Autodesk Inventor part; units mm, degrees
ref_plane "YZ Plane" through (0, 0, 0) normal (1, 0, 0) x (0, 1, 0)
ref_plane "XZ Plane" through (0, 0, 0) normal (0, 1, 0) x (-1, 0, 0)
ref_plane "XY Plane" through (0, 0, 0) normal (0, 0, 1) x (1, 0, 0)
sketch "Esboço1" plane through (0, 0, 0) normal (0, 1, 0) x (-1, 0, 0)
  line L0 (0, 0) -> (-91, 0)
  line L1 (-91, 0) -> (-91, -111)
  line L2 (-91, -111) -> (0, -111)
  line L3 (0, -111) -> (0, 0)
  line L4 (-3, -108) -> (-88, -108)
  line L5 (-88, -108) -> (-88, -3)
  line L6 (-88, -3) -> (-3, -3)
  line L7 (-3, -3) -> (-3, -108)
  dimension "d0" = 3
  dimension "d1" = 3
  dimension "d2" = 3
  dimension "d3" = 3
  dimension "d4" = 85
  dimension "d5" = 105
extrude "Extrusão1" add sketch "Esboço1" along normal blind 3 contours L4 L5 L6 L7
extrude "Extrusão2" add sketch "Esboço1" along normal blind 25
sketch "Esboço2" plane through (0, 0, 0) normal (0, 0, 1) x (1, 0, 0)
  circle A0 centre (20, 12) radius 3
  circle A1 centre (66, 13) radius 3.75
  line L0 (0, 0) -> (0, 25)
  line L1 (91, 0) -> (91, 25)
  line L2 (0, 0) -> (91, 0)
  point P0 (0, 12.5)
  dimension "d10" = 6
  dimension "d11" = 7.5
  dimension "d25" = 20
  dimension "d26" = 25
  dimension "d30" = 13
  dimension "d31" = 12
extrude "Extrusão3" cut sketch "Esboço2" against normal blind 30
sketch "Esboço3" plane through (91, 0, 0) normal (1, 0, 0) x (0, 0, -1)
  circle A0 centre (16.1671, 10) radius 1.5
  circle A1 centre (34.0898, 10) radius 1.5
  circle A2 centre (25.3707, 10) radius 1.5
  line L0 (0, 0) -> (111, 0)
  dimension "d14" = 3
  dimension "d15" = 3
  dimension "d16" = 3
  dimension "d32" = 10
  dimension "d33" = 10
  dimension "d34" = 10
extrude "Extrusão4" cut sketch "Esboço3" against normal blind 10
sketch "Esboço4" plane through (0, 3, 0) normal (0, 1, 0) x (1, 0, 0)
  line L0 (28.1, 81.6) -> (63, 81.6)
  line L1 (63, 81.6) -> (63, 98)
  line L2 (63, 98) -> (28.1, 98)
  line L3 (28.1, 98) -> (28.1, 81.6)
  line L4 (88, 108) -> (88, 3)
  line L5 (3, 108) -> (88, 108)
  point P0 (0, 0)
  point P1 (63, 89.8)
  dimension "d19" = 34.9
  dimension "d20" = 16.4
  dimension "d23" = 25
  dimension "d24" = 10
extrude "Extrusão5" cut sketch "Esboço4" against normal blind 1.5
properties part number "Caixa_3DPrint"
Work out the finished part from the listing and answer in its coordinate system (mm). A direction names the side the tool comes from. Coordinates: 2 decimals unless noted, no trailing zeros. Loops run counter-clockwise (first coordinate to the right, second up) from the corner with the lowest first, then second, coordinate; pieces in that order, holes last. Notation, with made-up numbers: M -34.5,3 L -12.5,3 A30 cw -12.5,26 Z; hole C 52.5,35 d3. An arc over 180 degrees is marked long. Answer in a Markdown table with one row per item. Add a question column.
1. Find section B-B, the plane y = 18.25. Write down the section's boundary in (x, z), then the cut area to 3 significant figures.
2. Find section C-C, the plane z = -94. Write down the section's boundary in (x, y), then the cut area to 3 significant figures.
3. Find section A-A, the plane x = 20. Write down the section's boundary in (y, z), then the cut area to 3 significant figures.
4. A tool of negligible diameter and unlimited length cuts with its end or side. For faces 5 (the cylindrical face through (69.577, 14.126, -1.479)), 6 (the flat face through (46, 12, -111)), 7 (the flat face through (46, 3, -55)), 8 (the cylindrical face through (89.52, 10.45, -17.6)), 9 (the flat face through (90, 25, -55)), from which of +Z, -Z, +X, -X, +Y, -Y can it reach the whole face along a straight path? Write none if from no direction.
5. The mould has two halves that part along X. Classify faces 1 (the flat face through (45, 1.5, -90)), 2 (the flat face through (91, 12, -55)), 3 (the cylindrical face through (89.521, 10.066, -23.872)), 4 (the flat face through (3, 14, -55)): pulls with the +X half, pulls with the -X half, needs draft (parallel to the pull), parting line crosses it, or undercut.
6. Find section D-D, the plane x = 48. Write down the section's boundary in (y, z), then the cut area to 3 significant figures.
7. Flat-ended cylindrical pins translate along their axes: P1, Ø4.5, axis at x = 66, y = 13, coming from the +Z side; P2, Ø8, axis at x = 40.5, z = -90, coming from the +Y side; P3, Ø8, axis at x = 51.5, z = -83.5, coming from the +Y side. Find the tip coordinate at first contact, or state that the pin passes through.
8. Consider L1, parallel to X at y = 13, z = -23; L2, parallel to Z at x = 44.5, y = 15.5; L3, parallel to Y at x = 66, z = -0.7. Determine where each line is inside the solid, lowest interval first.
Reported:
| question | item | result |
|---|---|---|
| 1 | outline | M 0,-111 L 91,-111 L 91,0 L 0,0 Z; hole M 3,-108 L 88,-108 L 88,-3 L 3,-3 Z |
| 1 | area | 1,180 mm^2 |
| 2 | outline | M 0,0 L 91,0 L 91,25 L 88,25 L 88,3 L 63,3 L 63,1.5 L 28.1,1.5 L 28.1,3 L 3,3 L 3,25 L 0,25 Z |
| 2 | area | 353 mm^2 |
| 3 | outline | M 0,-111 L 25,-111 L 25,-108 L 3,-108 L 3,-3 L 9,-3 L 9,0 L 0,0 Z; M 15,-3 L 25,-3 L 25,0 L 15,0 Z |
| 3 | area | 447 mm^2 |
| 4 | face 5 | +Z |
| 4 | face 6 | -Z, +X, -X, +Y, -Y |
| 4 | face 7 | +Y |
| 4 | face 8 | +X |
| 4 | face 9 | +Z, -Z, +X, -X, +Y |
| 5 | face 1 | undercut |
| 5 | face 2 | pulls with the +X half |
| 5 | face 3 | needs draft |
| 5 | face 4 | undercut |
| 6 | outline | M 0,-111 L 25,-111 L 25,-108 L 3,-108 L 3,-98 L 1.5,-98 L 1.5,-81.6 L 3,-81.6 L 3,-3 L 25,-3 L 25,0 L 0,0 Z |
| 6 | area | 440 mm^2 |
| 7 | P1 | stops at z = -108 |
| 7 | P2 | stops at y = 1.5 |
| 7 | P3 | stops at y = 3 |
| 8 | L1 | x = 0 to 3, 88 to 91 |
| 8 | L2 | z = -111 to -108, -3 to 0 |
| 8 | L3 | y = 0 to 9.25, 16.75 to 25 |
